Check sheet for the modelled part. Datum: model origin and axes. Units: mm. Give positions to 0.01 mm unless a question says otherwise; leave off trailing zeros. Loops run counter-clockwise (first coordinate to the right, second up) from the corner with the lowest first, then second, coordinate; pieces in that order, holes last. Notation, with made-up numbers: M 12,-25.75 L 59,-25.75 A11 ccw 59,-15.75 Z; hole C 59.5,-8.75 d7. An arc over 180 degrees is marked long. Write each question's results on one line, items separated by ' | '. Start each with the question number.
1. Go/stop test with flat-tipped pins: pin 1 (1.5 mm diameter, centred on y = 0.5, z = -1, fed in from -X); pin 2 (2.5 mm diameter, centred on y = 3, z = 2, fed in from -X); pin 3 (2.5 mm diameter, centred on y = 3, z = 2.5, fed in from +X); pin 4 (1.2 mm diameter, centred on x = 7, y = 3, fed in from -Z). Record where each tip stops, or that it passes through.
2. Sectioned sample at A-A on x = 14.25. Record the cut outline in (y, z), and give its area (3 significant figures).
3. Sectioned sample at D-D on y = 2.1. Record the cut outline in (x, z), and give its area (3 significant figures).
4. Sectioned sample at B-B on z = -0.65. Record the cut outline in (x, y).
5. Sectioned sample at C-C on y = 1.35. Record the cut outline in (x, z).
6. Material ranges on line 1 along Z through (x, y) = (11.75, 0.75); line 2 along X through (y, z) = (0.6, 0.7), recorded low to high.
```python
from build123d import *

# Parameters (mm, degrees)
SKETCH1_W           = 15.1
SKETCH1_H           = 4.2
BOSS_EXTRUDE1_DEPTH = 3.3
SKETCH5_R           = 0.3
FILLET1_R           = 0.15


with BuildPart() as part:
    # Sketch1 → Boss-Extrude1 (new body)
    with BuildSketch(Plane.XY):
        with Locations((7.55, 2.1)):
            Rectangle(SKETCH1_W, SKETCH1_H)
    extrude(amount=BOSS_EXTRUDE1_DEPTH)

    # Sweep3: sweep along a path in Sketch2
    with BuildLine(Plane(origin=(0, 2.1, 0), x_dir=(1, 0, 0), z_dir=(0, 1, 0))) as sweep3_path:
        Line((16.44, 1.8), (16.44, -0.9))
        ThreePointArc((16.44, -0.9), (16.220330086, -1.430330086), (15.69, -1.65))
        Line((15.69, -1.65), (15.1, -1.65))
        Line((15.1, -1.65), (0, -1.65))
        Line((0, -1.65), (-0.59, -1.65))
        ThreePointArc((-0.59, -1.65), (-1.120330086, -1.430330086), (-1.34, -0.9))
        Line((-1.34, -0.9), (-1.34, 1.8))
    # Sketch5 → Sweep3 (sweep)
    with BuildSketch(Plane.XY.offset(-1.8)):
        with Locations((-1.34, 2.1)):
            Circle(SKETCH5_R)
    sweep(path=sweep3_path.line)

    # Fillet1
    fillet1_edges = [part.edges().sort_by_distance(p)[0] for p in [
        (15.1, 2.1, 3.3),
        (7.55, 4.2, 3.3),
        (0, 2.1, 1.95),
        (15.1, 2.1, 1.95),
        (0, 2.1, 3.3),
        (7.55, 4.2, 0),
        (15.1, 2.1, 0),
        (7.55, 0, 0),
        (0, 2.1, 0),
        (7.55, 0, 3.3),
        (0, 4.2, 1.65),
        (15.1, 4.2, 1.65),
        (15.1, 0, 1.65),
        (0, 0, 1.65),
    ]]
    fillet(fillet1_edges, radius=FILLET1_R)


solid = part.part
```
Output values:
1) pin 1: through | pin 2: x = -1.62 | pin 3: x = 16.5 | pin 4: z = 0
2) outline: M 0,0.15 A0.15 ccw 0.15,0 L 4.05,0 A0.15 ccw 4.2,0.15 L 4.2,3.15 A0.15 ccw 4.05,3.3 L 0.15,3.3 A0.15 ccw 0,3.15 Z | area: 13.8 mm2
3) outline: M -1.64,-1.8 L -1.04,-1.8 L -1.04,0.9 A0.45 cw -0.59,1.35 L -0.15,1.35 A0.15 cw 0,1.2 L 0,0.15 A0.15 ccw 0.15,0 L 14.95,0 A0.15 ccw 15.1,0.15 L 15.1,1.2 A0.15 cw 15.25,1.35 L 15.69,1.35 A0.45 cw 16.14,0.9 L 16.14,-1.8 L 16.74,-1.8 L 16.74,0.9 A1.05 ccw 15.69,1.95 L 15.25,1.95 A0.15 cw 15.1,2.1 L 15.1,3.15 A0.15 ccw 14.95,3.3 L 0.15,3.3 A0.15 ccw 0,3.15 L 0,2.1 A0.15 cw -0.15,1.95 L -0.59,1.95 A1.05 ccw -1.64,0.9 Z | area: 55.2 mm2
4) outline: C -1.34,2.1 d0.6; C 16.44,2.1 d0.6
5) outline: M 0,0.15 A0.15 ccw 0.15,0 L 14.95,0 A0.15 ccw 15.1,0.15 L 15.1,3.15 A0.15 ccw 14.95,3.3 L 0.15,3.3 A0.15 ccw 0,3.15 Z
6) line 1: 0 to 3.3 | line 2: 0 to 15.1
